Read the model definition and answer for the solid it produces. Units are mm, in the model's axes. A direction names the side the tool comes from. Round coordinates to 2 decimals unless told otherwise and drop trailing zeros. Write each loop counter-clockwise with the first axis right and the second up, starting at its lowest first coordinate (ties: lowest second). Pieces come first, ordered by that corner, then holes. Notation, with made-up numbers: (83, 32.5) -> (112, 32.5) arc R24 ccw to (112, 55.5) -> close; hole circle Ø3 at (58, 42.5). An arc over 180 degrees is marked (long way). Return JSON: item names as keys, results as strings.
from build123d import *

# Parameters (mm, degrees)
F1_DEPTH = 457.2
F2_T     = 6.35
F3_W     = 205.1480994978
F3_H     = 457.2
F3_W_2   = 34.3874049749
F4_DEPTH = 6.35


with BuildPart() as f1:
    # F0 (on Front) → F1 (new body)
    with BuildSketch(Plane.XZ):
        Polygon((-127, 88.0205180943), (-127, -38.9794819057), (205.1480994978, -38.9794819057), align=None)
    extrude(amount=F1_DEPTH)

    # F2
    f2_openings = [f1.faces().sort_by_distance(p)[0] for p in [
        (-16.283967, -457.2, 3.353851),
        (-16.283967, 0, 3.353851),
    ]]
    offset(amount=F2_T, openings=f2_openings, kind=Kind.INTERSECTION)

    # F3 (on face) → F4 (cut)
    with BuildSketch(Plane(origin=(0, 0, -45.3294819057), x_dir=(1, 0, 0), z_dir=(0, 0, -1))):
        with Locations((102.5740497489, 228.6)):
            Rectangle(F3_W, F3_H)
        with Locations((222.3418019852, 228.6)):
            Rectangle(F3_W_2, F3_H)
    extrude(amount=-F4_DEPTH, mode=Mode.SUBTRACT)


solid = f1.part
Item 1: Section D-D (x = 143) is taken. Give the vertices of the cut face in (y, z).
Worked answers:
{"outline": "(-457.2, -15.22) -> (0, -15.22) -> (0, -8.42) -> (-457.2, -8.42) -> close"}
Item 2: Straight lines are drawn through the part: L1, parallel to Z at x = -28, y = -365.5; L2, parallel to Z at x = -81.5, y = -71; L3, parallel to Z at x = 91, y = -328. For each, find the intervals that lie inside material, in ascending order. Write a range as [from, to].
Worked answers:
{"L1": "z = [-45.33, -38.98], [50.17, 56.97]", "L2": "z = [-45.33, -38.98], [70.62, 77.42]", "L3": "z = [4.67, 11.46]"}
Item 3: Section B-B (x = -34) is taken. Give the vertices of the cut face in (y, z).
Worked answers:
{"outline": "(-457.2, -45.33) -> (0, -45.33) -> (0, -38.98) -> (-457.2, -38.98) -> close; (-457.2, 52.46) -> (0, 52.46) -> (0, 59.26) -> (-457.2, 59.26) -> close"}
Item 4: Flat-ended cylindrical pins translate along their axes: pin 1 (10 mm diameter, centred on x = 71.5, y = -294.5, fed in from -Z); pin 2 (12 mm diameter, centred on x = -61.5, z = 79.5, fed in from -Y); pin 3 (5 mm diameter, centred on x = 186.5, y = -391.5, fed in from -Z); pin 4 (7 mm diameter, centred on y = -245.5, z = -43, fed in from +X). Find the tip coordinate at first contact, or state that the pin passes through.
Worked answers:
{"pin 1": "stops at z = 10.21", "pin 2": "passes through", "pin 3": "stops at z = -32.81", "pin 4": "stops at x = 0"}
Item 5: Section C-C (y = -163) is taken. Give the vertices of the cut face in (x, z), then the cut area to 3 significant figures.
Worked answers:
{"outline": "(-133.35, -45.33) -> (0, -45.33) -> (0, -38.98) -> (-127, -38.98) -> (-127, 88.02) -> (205.15, -38.98) -> (222.93, -38.98) -> (-133.35, 97.25) -> close", "area": "4,020 mm2"}
Item 6: For a pull along Z with two mould halves and no side action, classify faces 1 (the flat face through (-127, -225, 25)), 2 (the flat face through (-22, 0, 53)), 3 (the flat face through (41.4, -225.4, 23.63)), 4 (the flat face through (47.28, -225.4, 28.18)) as released by +Z, released by -Z, zero draft, split by the parting line, or undercut.
Worked answers:
{"face 1": "undercut", "face 2": "zero draft", "face 3": "undercut", "face 4": "released by +Z"}
Item 7: Section A-A (z = 23) is taken. Give the vertices of the cut face in (x, y).
Worked answers:
{"outline": "(-133.35, -457.2) -> (-127, -457.2) -> (-127, 0) -> (-133.35, 0) -> close; (43.05, -457.2) -> (60.83, -457.2) -> (60.83, 0) -> (43.05, 0) -> close"}
Item 8: A tool of negligible diameter and unlimited length cuts with its end or side. For faces 5 (the flat face through (-64, -225, -38.979)), 6 (the flat face through (-22, -457.2, 53)), 7 (the flat face through (214, -232, -38.979)), from which of +Z, -Z, +X, -X, +Y, -Y can it reach the whole face along a straight path? Write none if from no direction.
Worked answers:
{"face 5": "+Y, -Y", "face 6": "+Z, -Z, +X, -X, -Y", "face 7": "-Z, +X, +Y, -Y"}
